Part model, mm, in its own coordinate system. A direction names the side the tool comes from. Coordinates: 2 decimals unless noted, no trailing zeros. Answer in a Markdown table with one row per item. Add a question column.
from build123d import *

# Parameters (mm, degrees)
SKETCH1_W               = 60
SKETCH1_H               = 60
BOSS_EXTRUDE1_DEPTH     = 90
SKETCH2_R               = 2
CUT_EXTRUDE1_DEPTH      = 10
MIRROR2_COPY_1_SKETCH_R = 2
MIRROR2_COPY_1_DEPTH    = 10


with BuildPart() as part:
    # Sketch1 → Boss-Extrude1 (new body)
    with BuildSketch(Plane(origin=(0, 0, 0), x_dir=(1, 0, 0), z_dir=(0, 1, 0))):
        Rectangle(SKETCH1_W, SKETCH1_H)
    extrude(amount=BOSS_EXTRUDE1_DEPTH)

    # Sketch2 → Cut-Extrude1 (cut)
    with BuildSketch(Plane(origin=(0, 90, 0), x_dir=(1, 0, 0), z_dir=(0, 1, 0))):
        with Locations((-25, 25)):
            Circle(SKETCH2_R)
    cut_extrude1 = extrude(amount=-CUT_EXTRUDE1_DEPTH, mode=Mode.SUBTRACT)

    # Mirror1: Cut-Extrude1 across plane
    add(cut_extrude1.mirror(Plane(origin=(0, 0, 0), x_dir=(0, 0, 1), z_dir=(1, 0, 0))), mode=Mode.SUBTRACT)

    # Mirror2: Cut-Extrude1 across plane
    add(cut_extrude1.mirror(Plane.XY), mode=Mode.SUBTRACT)

    # Mirror2 copy 1 sketch → Mirror2 copy 1 (cut)
    with BuildSketch(Plane(origin=(0, 90, 0), x_dir=(-1, 0, 0), z_dir=(0, 1, 0))):
        with Locations((-25, 25)):
            Circle(MIRROR2_COPY_1_SKETCH_R)
    extrude(amount=-MIRROR2_COPY_1_DEPTH, mode=Mode.SUBTRACT)


solid = part.part
(1) Drop a flat-ended pin along its axis: P1, Ø2.5, axis at x = 25, z = 25, coming from the +Y side. Give the stop position or say it passes through.
(2) Pull direction Z, two halves, no side cores. Call faces 1 (the flat face through (0, 44, -30)), 2 (the flat face through (25, 80, -25)), 3 (the cylindrical face through (-26.6, 85.1, -23.8)), 4 (the flat face through (-30, 44, 0)): pulls with the +Z half, pulls with the -Z half, needs draft (parallel to the pull), parting line crosses it, or undercut.
(3) 3-axis set-ups, long thin cutter, end or side, ignore diameter. For faces 5 (the flat face through (0, 0, 0)), 6 (the cylindrical face through (26.6, 85.1, 23.8)): which of +Z, -Z, +X, -X, +Y, -Y reach the whole face in a straight line?
(4) Wall check: line 1 (X direction, y = 85, z = -25). Give the ranges that are in metal, low to high.
Computed:
| question | item | result |
|---|---|---|
| 1 | P1 | stops at y = 80 |
| 2 | face 1 | pulls with the -Z half |
| 2 | face 2 | undercut |
| 2 | face 3 | undercut |
| 2 | face 4 | needs draft |
| 3 | face 5 | +Z, -Z, +X, -X, -Y |
| 3 | face 6 | +Y |
| 4 | line 1 | x = -30 to -27, -23 to 23, 27 to 30 |
